```python
from build123d import *
from OCP.BRepFilletAPI import BRepFilletAPI_MakeChamfer

# Parameters (mm, degrees)
SKIZZE1_W                            = 120
SKIZZE1_H                            = 22
AUFSATZ_LINEAR_AUSTRAGEN1_DEPTH      = 22
SCHNITT_LINEAR_AUSTRAGEN1_DEPTH      = 124.967737738
SCHNITT_LINEAR_AUSTRAGEN1_DEPTH_BACK = 124.967737738
SCHNITT_LINEAR_AUSTRAGEN5_DEPTH      = 124.967737738
SCHNITT_LINEAR_AUSTRAGEN6_DEPTH      = 124.967737738
VERRUNDUNG1_R                        = 2
SCHNITT_LINEAR_AUSTRAGEN7_DEPTH      = 73.062472897
KREISMUSTER1_COUNT                   = 4
FASE1_SIZE                           = 1
FASE1_SIZE2                          = 1.022482955
SCHNITT_LINEAR_AUSTRAGEN8_DEPTH      = 10


with BuildPart() as part:
    # Skizze1 → Aufsatz-Linear austragen1 (new body)
    with BuildSketch(Plane.XY):
        with Locations((60, 11)):
            Rectangle(SKIZZE1_W, SKIZZE1_H)
    extrude(amount=AUFSATZ_LINEAR_AUSTRAGEN1_DEPTH)

    # Skizze2 → Schnitt-Linear austragen1 (cut, two sides: drawn at the far end of the back side and taken through both)
    with BuildSketch(Plane(origin=(0, 22, 0), x_dir=(1, 0, 0), z_dir=(0, 1, 0)).offset(-SCHNITT_LINEAR_AUSTRAGEN1_DEPTH_BACK)):
        Polygon((120, -11), (65, -22), (120, -22), align=None)
    extrude(amount=SCHNITT_LINEAR_AUSTRAGEN1_DEPTH + SCHNITT_LINEAR_AUSTRAGEN1_DEPTH_BACK, mode=Mode.SUBTRACT)

    # Skizze3 → Schnitt-Linear austragen5 (cut, through all)
    with BuildSketch(Plane.XZ):
        Polygon((120, 11), (65, 0), (120, 0), align=None)
    extrude(amount=-SCHNITT_LINEAR_AUSTRAGEN5_DEPTH, mode=Mode.SUBTRACT)

    # Skizze5 → Schnitt-Linear austragen6 (cut, through all)
    with BuildSketch(Plane(origin=(0, 0, 0), x_dir=(-1, 0, 0), z_dir=(0, 0, -1))):
        with BuildLine():
            Line((-54, 18.5), (-40, 18.5))
            ThreePointArc((-40, 18.5), (-32.5, 11), (-40, 3.5))
            Line((-40, 3.5), (-54, 3.5))
            ThreePointArc((-54, 3.5), (-61.5, 11), (-54, 18.5))
        make_face()
    extrude(amount=-SCHNITT_LINEAR_AUSTRAGEN6_DEPTH, mode=Mode.SUBTRACT)

    # Verrundung1
    verrundung1_edges = [part.edges().sort_by_distance(p)[0] for p in [
        (120, 11, 11),
    ]]
    fillet(verrundung1_edges, radius=VERRUNDUNG1_R)

    # 3D-Skizze1 → Schnitt-Linear austragen7 (cut, through all)
    with BuildSketch(Plane(origin=(65, 22, 22), x_dir=(-0.9995269630766537, 0, -0.03075467578697402), z_dir=(-0.02175198393938513, 0.7069394780300152, 0.7069394780300153))):
        Polygon((0, 0), (65.030761952, 0), (64.9692526, 2.827758229), align=None)
    schnitt_linear_austragen7 = extrude(amount=SCHNITT_LINEAR_AUSTRAGEN7_DEPTH, mode=Mode.SUBTRACT)

    # Kreismuster1: Schnitt-Linear austragen7 ×4 about axis
    kreismuster1_axis = Axis((0, 10.957123098, 10.957123098), (1, 0, 0))
    for i in range(1, KREISMUSTER1_COUNT):
        add(schnitt_linear_austragen7.rotate(kreismuster1_axis, i * 360 / KREISMUSTER1_COUNT), mode=Mode.SUBTRACT)

    # Fase1: one chamfer whose edges measure the first distance from different faces: ONE call of the kernel's chamfer builder (chamfer() names one face for all edges)
    fase1_edges_1 = [part.edges().sort_by_distance(p)[0] for p in [
        (0, 21, 21),
        (0, 0.957123098, 21.042876902),
        (0, 0.914246196, 0.914246196),
        (0, 21.042876902, 0.957123098),
    ]]
    fase1_side_1 = [part.faces().sort_by_distance(p)[0] for p in [
        (0, 10.993083294, 10.993083294),
    ]]
    fase1_edges_2 = [part.edges().sort_by_distance(p)[0] for p in [
        (0, 10.957123098, 22),
        (0, 0, 10.957123098),
        (0, 10.957123098, 0),
        (0, 22, 10.957123098),
    ]]
    fase1 = BRepFilletAPI_MakeChamfer(part.part.solid().wrapped)
    for e in fase1_edges_1:
        fase1.Add(FASE1_SIZE, FASE1_SIZE2, e.wrapped, fase1_side_1[0].wrapped)  # the first distance lies on this face
    for e in fase1_edges_2:
        fase1.Add(FASE1_SIZE, e.wrapped)
    add(Compound.cast(fase1.Shape()), mode=Mode.REPLACE)

    # Skizze6 → Schnitt-Linear austragen8 (cut)
    with BuildSketch(Plane.ZY):
        with BuildLine():
            Line((12.621096819, 12.381864671), (12.35186605, 12.126656338))
            add(Edge.make_bspline(
                [(12.35186605, 12.126656338), (12.303147162, 12.172487201), (12.206871115, 12.263056064), (12.049910873, 12.380567059), (11.886147239, 12.481233159), (11.716434742, 12.563139395), (11.544976188, 12.628492156), (11.374047412, 12.675020296), (11.20540171, 12.704692834), (11.093234492, 12.708241203), (11.037963806, 12.709989671)],
                knots=[0, 0, 0, 0, 1.08915593, 2.152340314, 3.188132944, 4.216796309, 5.218260357, 6.173443236, 7.099959455, 8, 8, 8, 8], degree=3))
            add(Edge.make_bspline(
                [(11.037963806, 12.709989671), (11.004049107, 12.709576065), (10.936307666, 12.708749926), (10.835685722, 12.698205711), (10.736119085, 12.683040847), (10.63779571, 12.661098969), (10.540524424, 12.63328991), (10.444643531, 12.598504446), (10.349974177, 12.557949202), (10.257408096, 12.511086728), (10.167667592, 12.459606882), (10.082910757, 12.402558341), (10.002597358, 12.341769551), (9.928236932, 12.275718572), (9.859401746, 12.205003707), (9.794453374, 12.1309404), (9.735676078, 12.051505182), (9.682584913, 11.968159556), (9.635223294, 11.882367367), (9.593414641, 11.794954377), (9.558317553, 11.706210523), (9.530548098, 11.616024445), (9.507637444, 11.525093855), (9.491519836, 11.432789134), (9.482433114, 11.339011449), (9.480861334, 11.276214191), (9.480071178, 11.24464512)],
                knots=[0, 0, 0, 0, 1.02818874, 2.053710826, 3.065248034, 4.081641283, 5.106893873, 6.131558223, 7.173050175, 8.228653731, 9.27666206, 10.308777013, 11.325269123, 12.329503258, 13.32196095, 14.316845687, 15.314881793, 16.315733098, 17.311955233, 18.285320748, 19.252783886, 20.203351036, 21.145449891, 22.095197417, 23.042428769, 24, 24, 24, 24], degree=3))
            add(Edge.make_bspline(
                [(9.480071178, 11.24464512), (9.480826897, 11.212374302), (9.482336269, 11.147920789), (9.491996589, 11.051726716), (9.509924829, 10.956961314), (9.533892538, 10.863313181), (9.563873354, 10.770621933), (9.60124602, 10.679289423), (9.645511621, 10.589319032), (9.696748173, 10.501521415), (9.752934376, 10.415998392), (9.815877457, 10.33543887), (9.88273804, 10.258770093), (9.95595194, 10.187694329), (10.033171483, 10.120310432), (10.116703759, 10.058474911), (10.204906219, 10.000996687), (10.297913431, 9.948600168), (10.394716213, 9.901791632), (10.493972966, 9.860167736), (10.596000782, 9.825888399), (10.700263472, 9.797950295), (10.806636743, 9.775049998), (10.915660546, 9.760317517), (11.026533254, 9.749626686), (11.101271887, 9.748845016), (11.138925345, 9.748451209)],
                knots=[0, 0, 0, 0, 0.93586088, 1.869166235, 2.799637598, 3.729985548, 4.670839027, 5.622275134, 6.589130586, 7.576015415, 8.568469353, 9.55398029, 10.53834874, 11.515998671, 12.510579167, 13.508179873, 14.527009472, 15.561807829, 16.601455013, 17.643573243, 18.680854198, 19.719860599, 20.772568776, 21.833555941, 22.908541556, 24, 24, 24, 24], degree=3))
            add(Edge.make_bspline(
                [(11.138925345, 9.748451209), (11.184303692, 9.749399786), (11.273411449, 9.751262469), (11.404397892, 9.765762759), (11.530200963, 9.788409553), (11.650467166, 9.821575449), (11.765336187, 9.863879124), (11.875229128, 9.914874511), (11.979280787, 9.97651757), (12.07780396, 10.046091437), (12.168561146, 10.123606269), (12.25041527, 10.207250724), (12.322060759, 10.296618791), (12.384565458, 10.391184106), (12.436274113, 10.491729411), (12.478716908, 10.597761974), (12.511250199, 10.709329486), (12.524605174, 10.786421118), (12.53135323, 10.825374286)],
                knots=[0, 0, 0, 0, 1.13008108, 2.219097802, 3.278683437, 4.311054135, 5.322181354, 6.324827112, 7.324222904, 8.330512327, 9.32562643, 10.293043162, 11.24128371, 12.174520618, 13.111833804, 14.052305215, 15.015860969, 16, 16, 16, 16], degree=3))
            Line((12.53135323, 10.825374286), (11.364686563, 10.825374286))
            Line((11.364686563, 10.825374286), (11.364686563, 11.184348645))
            Line((11.364686563, 11.184348645), (12.845455794, 11.184348645))
            add(Edge.make_bspline(
                [(12.845455794, 11.184348645), (12.843749945, 11.117441157), (12.840411292, 10.986491115), (12.816992376, 10.795520844), (12.779175864, 10.615149151), (12.727515552, 10.445186079), (12.660640272, 10.285872486), (12.579267743, 10.13704662), (12.482095622, 9.999669939), (12.372585181, 9.872620936), (12.249685223, 9.759291723), (12.116716603, 9.659685785), (11.973459635, 9.57578317), (11.820049827, 9.507522508), (11.656989394, 9.454248513), (11.483901014, 9.416476936), (11.301019413, 9.393846973), (11.175682736, 9.390955593), (11.111581595, 9.38947685)],
                knots=[0, 0, 0, 0, 1.140356446, 2.231883559, 3.274166699, 4.278491846, 5.25512956, 6.21435461, 7.1637429, 8.11826594, 9.068280886, 10.0076534, 10.945064095, 11.891975133, 12.864533718, 13.863980011, 14.907571808, 16, 16, 16, 16], degree=3))
            add(Edge.make_bspline(
                [(11.111581595, 9.38947685), (11.07207146, 9.390045972), (10.994144739, 9.391168462), (10.879053811, 9.39914581), (10.76713619, 9.411426386), (10.658408181, 9.429971509), (10.552469839, 9.452686164), (10.449850254, 9.481772882), (10.350158512, 9.515441582), (10.253240526, 9.553737255), (10.15997598, 9.598108912), (10.069949463, 9.647418551), (9.982663337, 9.701411912), (9.898712172, 9.761022758), (9.81765855, 9.825805218), (9.740025107, 9.895889137), (9.665377229, 9.971060257), (9.618616765, 10.024439266), (9.595055153, 10.051335825)],
                knots=[0, 0, 0, 0, 1.107784379, 2.184907829, 3.233506516, 4.263428166, 5.276301166, 6.270063455, 7.25232949, 8.225834625, 9.190232166, 10.146266622, 11.1027726, 12.066435141, 13.031522626, 14.010570082, 14.99756817, 16, 16, 16, 16], degree=3))
            add(Edge.make_bspline(
                [(9.595055153, 10.051335825), (9.560869221, 10.094006478), (9.493064808, 10.178639495), (9.405786651, 10.314239439), (9.331385249, 10.4546413), (9.271017426, 10.600235928), (9.22387934, 10.750887141), (9.190073087, 10.906402432), (9.170265798, 11.066982063), (9.167412261, 11.175647327), (9.165968614, 11.230622684)],
                knots=[0, 0, 0, 0, 1.023165419, 2.029347347, 3.013907458, 3.994755782, 4.975994455, 5.96558838, 6.970761222, 8, 8, 8, 8], degree=3))
            add(Edge.make_bspline(
                [(9.165968614, 11.230622684), (9.166500852, 11.271788937), (9.167558564, 11.353598244), (9.18038408, 11.475055551), (9.198785498, 11.594356244), (9.225832553, 11.7114028), (9.259928818, 11.826273392), (9.302482304, 11.939021355), (9.3520272, 12.049713227), (9.409612696, 12.157587095), (9.473697155, 12.261211508), (9.543247376, 12.360169311), (9.619250976, 12.452658376), (9.700466775, 12.539850024), (9.787863766, 12.620648871), (9.880623189, 12.695802982), (9.978816532, 12.765413168), (10.082752712, 12.828383003), (10.190880396, 12.884946623), (10.302940398, 12.934535835), (10.418898509, 12.97551915), (10.537885986, 13.01029293), (10.660803487, 13.036008071), (10.786759024, 13.054656816), (10.916409136, 13.067417416), (11.004045165, 13.068443671), (11.048480633, 13.06896403)],
                knots=[0, 0, 0, 0, 1.008945113, 2.00506715, 2.99143336, 3.967273523, 4.948097931, 5.927297278, 6.919902385, 7.919676788, 8.923139349, 9.905703106, 10.883022732, 11.856032218, 12.825136022, 13.798837087, 14.781400844, 15.773989409, 16.776158564, 17.77167057, 18.775803737, 19.789618931, 20.80898985, 21.851988756, 22.910860228, 24, 24, 24, 24], degree=3))
            add(Edge.make_bspline(
                [(11.048480633, 13.06896403), (11.084718877, 13.068384538), (11.156575056, 13.067235474), (11.263500788, 13.059270826), (11.368773803, 13.046646945), (11.472550193, 13.029420158), (11.574476559, 13.005956468), (11.674843264, 12.977878183), (11.7737958, 12.945186361), (11.87102405, 12.906197514), (11.967181766, 12.861943889), (12.062803606, 12.812130467), (12.157562852, 12.755905462), (12.251623834, 12.693101927), (12.345579691, 12.624798509), (12.437944334, 12.549041685), (12.530947278, 12.46881893), (12.590749092, 12.411136746), (12.621096819, 12.381864671)],
                knots=[0, 0, 0, 0, 0.985871117, 1.954866573, 2.915460327, 3.869826059, 4.81536089, 5.759505086, 6.70452669, 7.649098992, 8.607881297, 9.583363685, 10.581137262, 11.603961102, 12.659522466, 13.73993555, 14.853081303, 16, 16, 16, 16], degree=3))
        make_face()
        Polygon((13.563404512, 12.97922044), (13.877507076, 12.97922044), (13.877507076, 9.838194799), (15.223660922, 9.838194799), (15.223660922, 9.47922044), (13.563404512, 9.47922044), align=None)
    extrude(amount=-SCHNITT_LINEAR_AUSTRAGEN8_DEPTH, mode=Mode.SUBTRACT)


solid = part.part
```
The listing builds one solid part. Answer for the finished solid, in the listing's coordinates (mm). A direction names the side the tool comes from. Round coordinates to 2 decimals unless told otherwise and drop trailing zeros. Loops run counter-clockwise (first coordinate to the right, second up) from the corner with the lowest first, then second, coordinate; pieces in that order, holes last.
Q1. Section D-D, the plane x = 94 is taken. Determine the outline of the cut face in (y, z), then the cut area to 3 significant figures.
Q2. For a pull along X with two mould halves and no side action, classify faces 1 (the face through (32.5, 11.16, 10.85)), 2 (the face through (111.8, 11.2, 11)), 3 (the face through (0, 11, 11)) as released by +X, released by -X, zero draft, split by the parting line, or undercut.
Q3. Section C-C, the plane z = 4.25 is taken. Determine the outline of the cut face in (x, y).
Q4. Section A-A, the plane y = 15.5 is taken. Determine the outline of the cut face in (x, z).
Q5. Find the intervals of material crossed by line 1 (Y direction, x = 39.5, z = 5.5); line 2 (X direction, y = 8.5, z = 12.5); line 3 (Z direction, x = 21.5, y = 1), in increasing order.
Q6. Section B-B, the plane x = 49 is taken. Determine the outline of the cut face in (y, z), then the cut area to 3 significant figures.
Q7. Which of the six approach directions +Z, -Z, +X, -X, +Y, -Y give full straight-line access (tool end or side, diameter ignored) to faces 4 (the face through (0.52, 20.69, 1.28)), 5 (the face through (10, 11, 12)), 6 (the face through (47, 18.5, 11))?
Completed:
1. outline: (0, 5.8) - (22, 5.8) - (22, 16.2) - (0, 16.2) - close
1. area: 229 mm2
2. face 1: undercut
2. face 2: released by +X
2. face 3: released by -X
3. outline: (0, 1) - (1, 0) - (86.25, 0) - (86.25, 22) - (1, 22) - (0, 21) - close; hole (40, 3.5) - (54, 3.5) arc R7.5 ccw to (54, 18.5) - (40, 18.5) arc R7.5 ccw to start
4. outline: (0, 1) - (1, 0) - (34, 0) - (34, 22) - (1, 22) - (0, 21) - close; (60, 0) - (65, 0) - (110.19, 9.04) arc R2 ccw to (110.19, 12.96) - (65, 22) - (60, 22) - close
5. line 1: y = 0 to 3.52, 18.48 to 22
5. line 2: x = 0 to 32.93, 61.07 to 111.12
5. line 3: z = 0.17 to 21.75
6. outline: (0, 0.32) - (0.32, 0) - (3.5, 0) - (3.5, 22) - (0.41, 22) - (0, 21.59) - close; (18.5, 0) - (21.59, 0) - (22, 0.41) - (22, 21.51) - (21.51, 22) - (18.5, 22) - close
6. area: 154 mm2
7. face 4: -Z, -X, +Y
7. face 5: -X
7. face 6: +Z, -Z
